Could you check a few things on this model? Use its own coordinates, in mm. Coordinates: 2 decimals unless noted, no trailing zeros. Order: outer loops, then holes, each group sorted by start corner. A loop starts at its lowest first (then second) coordinate and runs counter-clockwise, first axis right, second up.
Autodesk Inventor part; units mm, degrees
ref_plane "YZ Plane" through (0, 0, 0) normal (1, 0, 0) x (0, 1, 0)
ref_plane "XZ Plane" through (0, 0, 0) normal (0, 1, 0) x (-1, 0, 0)
ref_plane "XY Plane" through (0, 0, 0) normal (0, 0, 1) x (1, 0, 0)
sketch "Sketch1" plane through (0, 0, 0) normal (0, 0, 1) x (1, 0, 0)
  line L0 (-145, -145) -> (145, -145)
  line L1 (145, -145) -> (145, 145)
  line L2 (145, 145) -> (-145, 145)
  line L3 (-145, 145) -> (-145, -145)
  line L4 (-145, -145) -> (145, 145) construction
  line L5 (145, -145) -> (-145, 145) construction
  point P0 (0, 0)
  dimension "d0" = 290
  dimension "d1" = 290
extrude "Extrusion1" add sketch "Sketch1" along normal blind 5
sketch "Sketch2" plane through (0, 0, 5) normal (0, 0, 1) x (1, 0, 0)
  point P0 (0, 0)
  point P1 (0, 0)
hole "Hole1" at (0, 0, 5) direction (0, 0, -1) diameter 6.6 depth 8 tip angle 118
sketch "Sketch3" plane through (0, 0, 5) normal (0, 0, 1) x (1, 0, 0)
  line L0 (-137.5, -137.5) -> (137.5, -137.5) construction
  line L1 (137.5, -137.5) -> (137.5, 137.5) construction
  line L2 (137.5, 137.5) -> (-137.5, 137.5) construction
  line L3 (-137.5, 137.5) -> (-137.5, -137.5) construction
  line L4 (-137.5, -137.5) -> (137.5, 137.5) construction
  line L5 (137.5, -137.5) -> (-137.5, 137.5) construction
  point P0 (0, 0)
  dimension "d11" = 275
  dimension "d12" = 275
hole "Hole2" at (-137.5, 137.5, 5) at (137.5, 137.5, 5) at (137.5, -137.5, 5) at (-137.5, -137.5, 5) direction (0, 0, -1) diameter 5.5 depth 8 tip angle 118
fillet "Fillet1" radius 6 4 edges at (-145, -145, 2.5) (145, -145, 2.5) (145, 145, 2.5) (-145, 145, 2.5)
sketch "Sketch4" plane through (0, 0, 5) normal (0, 0, 1) x (1, 0, 0)
  line L0 (-120, -140) -> (120, -140)
  line L1 (120, -140) -> (120, -135)
  line L2 (120, -135) -> (-120, -135)
  line L3 (-120, -135) -> (-120, -140)
  line L4 (140, -120) -> (135, -120)
  line L5 (135, -120) -> (135, 120)
  line L6 (135, 120) -> (140, 120)
  line L7 (140, 120) -> (140, -120)
  line L8 (120, 141) -> (-120, 141)
  line L9 (-120, 141) -> (-120, 136)
  line L10 (-120, 136) -> (120, 136)
  line L11 (120, 136) -> (120, 141)
  line L12 (-135, 120) -> (-140, 120)
  line L13 (-140, 120) -> (-140, -120)
  line L14 (-140, -120) -> (-135, -120)
  line L15 (-135, -120) -> (-135, 120)
  line L16 (-139, -145) -> (139, -145)
  line L17 (145, -139) -> (145, 139)
  line L18 (139, 145) -> (-139, 145)
  line L19 (-145, 139) -> (-145, -139)
  point P0 (0, 0)
  point P1 (0, 136)
  point P2 (-135, 0)
  dimension "d21" = 5
  dimension "d22" = 5
  dimension "d23" = 240
  dimension "d24" = 240
  dimension "d25" = 5
  dimension "d26" = 5
  dimension "d27" = 5
  dimension "d28" = 5
  dimension "d29" = 4
  dimension "d30" = 5
extrude "Extrusion2" cut sketch "Sketch4" against normal through all
sketch "Sketch5" plane through (0, 0, 5) normal (0, 0, 1) x (1, 0, 0)
  point P0 (0, 0)
  point P1 (-120, 0)
  point P2 (120, 120)
  dimension "d34" = 120
  dimension "d51" = 120
  dimension "d52" = 120
hole "Hole3" at (-120, 0, 5) at (120, 120, 5) direction (0, 0, -1) diameter 12 depth 8 tip angle 118
sketch "Sketch6" plane through (0, 0, 5) normal (0, 0, 1) x (1, 0, 0)
  point P0 (0, 0)
  point P1 (0, 120)
  dimension "d50" = 120
hole "Hole4" at (0, 120, 5) direction (0, 0, -1) diameter 8 depth 8 tip angle 118
properties part number "Main" material "Polycarbonate, Clear"
Item 1: For pin 1 Ø4 at (x, y) = (0, 0) entering from -Z, with a flat end and sliding along its axis, tell me the tip position at first contact or that it passes through.
Item 2: Suppose I cut it at B-B (y = -95). List the corners of the cut face in (x, z) for me.
Item 3: Thinking about a two-plate mould opening in Y: for faces 1 (the face through (30, 2, 0)), 2 (the face through (1.532, 116.305, 2.465)), which applies, +Y half, -Y half, draft (parallel to the pull), parting line (faces both ways), or undercut?
Item 4: Suppose I cut it at C-C (z = 3.1). Count the separate pieces of the cut face and the enclosed holes in it, and give its area (3 significant figures).
Item 5: I need wall thicknesses on line 1 (X direction, y = 64.5, z = 3.5); line 2 (Y direction, x = 137.5, z = 3.1); line 3 (Y direction, x = 98, z = 2.05). Which ranges of each line are inside material? Lowest first, please.
Item 6: Suppose I cut it at D-D (x = -70). List the corners of the cut face in (y, z) for me.
Item 7: Suppose I cut it at A-A (y = 0). List the corners of the cut face in (x, z) for me, and give its area (3 significant figures).
Geometry results:
1. pin 1: passes through
2. outline: (-145, 0) - (-140, 0) - (-140, 5) - (-145, 5) - close; (-135, 0) - (135, 0) - (135, 5) - (-135, 5) - close; (140, 0) - (145, 0) - (145, 5) - (140, 5) - close
3. face 1: draft
3. face 2: undercut
4. separate pieces: 1
4. enclosed holes: 12
4. area: 78,900 mm2
5. line 1: x = -145 to -140, -135 to 135, 140 to 145
5. line 2: y = -145 to -140.25, -134.75 to -120, 120 to 134.75, 140.25 to 145
5. line 3: y = -145 to -140, -135 to 136, 141 to 145
6. outline: (-145, 0) - (-140, 0) - (-140, 5) - (-145, 5) - close; (-135, 0) - (136, 0) - (136, 5) - (-135, 5) - close; (141, 0) - (145, 0) - (145, 5) - (141, 5) - close
7. outline: (-145, 0) - (-140, 0) - (-140, 5) - (-145, 5) - close; (-135, 0) - (-126, 0) - (-126, 5) - (-135, 5) - close; (-114, 0) - (-3.3, 0) - (-3.3, 5) - (-114, 5) - close; (3.3, 0) - (135, 0) - (135, 5) - (3.3, 5) - close; (140, 0) - (145, 0) - (145, 5) - (140, 5) - close
7. area: 1,310 mm2
